```python
from build123d import *

# Parameters (mm, degrees)
F1_DEPTH = 4.8


# Not quite as in the source:
# - a feature names something its author has since deleted; it is built from what else it names


with BuildPart() as f1:
    # F0 (on Front) → F1 (new body)
    with BuildSketch(Plane.XZ):
        Polygon((-36.6599317901, 103.4564594077), (-174.1599317901, 103.4564594077), (-174.1599317901, 34.6020694077), (-174.1599317901, 29.6020694077), (-174.1599317901, 24.6020694077), (-174.1599317901, -56.5435405923), (-36.6599317901, -56.5435405923), (-36.6599317901, -23.3979305923), (-119.1599317901, -23.3979305923), (-119.1599317901, 82.6020694077), (-36.6599317901, 82.6020694077), align=None)
        Polygon((100.8400682099, 103.4564594077), (-36.6599317901, 103.4564594077), (-36.6599317901, 82.6020694077), (45.8400682099, 82.6020694077), (45.8400682099, -23.3979305923), (-36.6599317901, -23.3979305923), (-36.6599317901, -56.5435405923), (100.8400682099, -56.5435405923), (100.8400682099, 24.6020694077), (100.8400682099, 29.6020694077), (100.8400682099, 34.6020694077), align=None)
        Polygon((105.3400682099, 34.6020694077), (100.8400682099, 34.6020694077), (100.8400682099, 29.6020694077), (101.9359001704, 29.6020694077), (105.3400682099, 29.6020694077), align=None)
        Polygon((101.9359001704, 29.6020694077), (100.8400682099, 29.6020694077), (100.8400682099, 24.6020694077), (101.9359001704, 24.6020694077), (105.3400682099, 24.6020694077), (105.3400682099, 29.6020694077), align=None)
        Polygon((-174.1599317901, 29.6020694077), (-174.1599317901, 34.6020694077), (-178.6599317901, 34.6020694077), (-178.6599317901, 29.6020694077), (-175.2557637506, 29.6020694077), align=None)
        Polygon((-174.1599317901, 24.6020694077), (-174.1599317901, 29.6020694077), (-175.2557637506, 29.6020694077), (-178.6599317901, 29.6020694077), (-178.6599317901, 24.6020694077), (-175.2557637506, 24.6020694077), align=None)
    extrude(amount=F1_DEPTH)


solid = f1.part
```
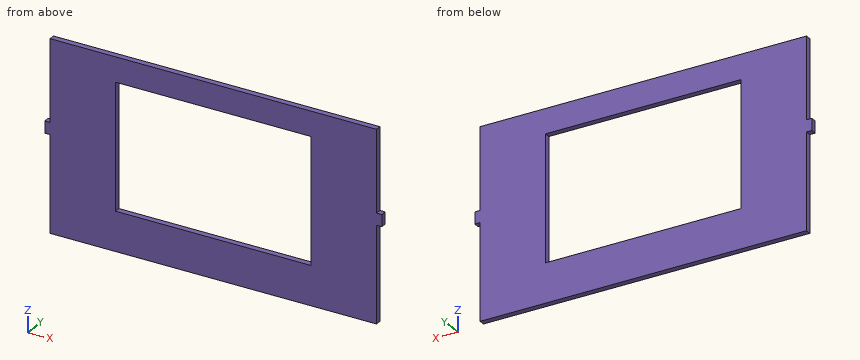
Here's how the part is built. I have some questions about the finished solid (model axes, mm). Give positions to 0.01 mm unless a question says otherwise; leave off trailing zeros. Loops run counter-clockwise (first coordinate to the right, second up) from the corner with the lowest first, then second, coordinate; pieces in that order, holes last. Notation, with made-up numbers: (71.5, 10.25) -> (80.5, 10.25) arc R28 ccw to (80.5, 47.25) -> close; hole circle Ø11 at (44, -35.75). An arc over 180 degrees is marked (long way). Use one line per item in the form item = value. Start each with the question number.
1) Imagine slicing it at D-D (z = -30.5). Please give me the cut outline in (x, y).
2) Imagine slicing it at B-B (z = 5). Please give me the cut outline in (x, y).
3) Imagine slicing it at C-C (y = -1). Please give me the cut outline in (x, z), then the cut area to 3 significant figures.
4) For P1, Ø2, axis at x = 103.5, y = -3, coming from the -Z side; P2, Ø1.4, axis at y = -1.5, z = 5, coming from the +X side; P3, Ø8, axis at x = -146, z = -16, coming from the +Y side; P4, Ø2.5, axis at y = -3, z = -8.5, coming from the -X side, each with a flat end and sliding along its axis, tell me the tip position at first contact or that it passes through.
5) Imagine slicing it at A-A (x = -68.5). Please give me the cut outline in (y, z).
6) Please list where these lines run through material, in increasing order: line 1 along X through (y, z) = (-2.6, -10.5); line 2 along Z through (x, y) = (-63, -3.3); line 3 along X through (y, z) = (-1.45, -24.5).
Check values:
q1.outline = (-174.16, -4.8) -> (100.84, -4.8) -> (100.84, 0) -> (-174.16, 0) -> close
q2.outline = (-174.16, -4.8) -> (-119.16, -4.8) -> (-119.16, 0) -> (-174.16, 0) -> close; (45.84, -4.8) -> (100.84, -4.8) -> (100.84, 0) -> (45.84, 0) -> close
q3.outline = (-178.66, 24.6) -> (-174.16, 24.6) -> (-174.16, -56.54) -> (100.84, -56.54) -> (100.84, 24.6) -> (105.34, 24.6) -> (105.34, 34.6) -> (100.84, 34.6) -> (100.84, 103.46) -> (-174.16, 103.46) -> (-174.16, 34.6) -> (-178.66, 34.6) -> close; hole (-119.16, -23.4) -> (45.84, -23.4) -> (45.84, 82.6) -> (-119.16, 82.6) -> close
q3.area = 26,600 mm^2
q4.P1 = 24.6
q4.P2 = 100.84
q4.P3 = 0
q4.P4 = -174.16
q5.outline = (-4.8, -56.54) -> (0, -56.54) -> (0, -23.4) -> (-4.8, -23.4) -> close; (-4.8, 82.6) -> (0, 82.6) -> (0, 103.46) -> (-4.8, 103.46) -> close
q6.line_1 = -174.16 to -119.16, 45.84 to 100.84
q6.line_2 = -56.54 to -23.4, 82.6 to 103.46
q6.line_3 = -174.16 to 100.84
